Geometry check sheet. Reference: the model listing, model coordinates, mm. Round coordinates to 2 decimals unless told otherwise and drop trailing zeros. Loops run counter-clockwise (first coordinate to the right, second up) from the corner with the lowest first, then second, coordinate; pieces in that order, holes last. Notation, with made-up numbers: (63, 35.5) -> (90, 35.5) arc R29 ccw to (90, 65.5) -> close; hole circle Ø7 at (59, 22). An arc over 180 degrees is marked (long way). Use a Markdown table: item, result. Add a question column.
Q1. Gauge pin test, flat end, axial feed: P1, Ø1, axis at x = 0.5, z = 2.5, coming from the -Y side. Record the tip position at first contact, or that the pin passes through.
Q2. Sectioned sample at B-B, the plane x = 4.5. Enter the section's corners in (y, z).
Q3. Sectioned sample at A-A, the plane y = -6. Enter the section's corners in (x, z).
Q4. Material ranges on L1, parallel to Y at x = 2.75, z = 2.2; L2, parallel to X at y = -1.5, z = 4.25, recorded low to high.
```python
from build123d import *

# Parameters (mm, degrees)
F0_R     = 10
F1_DEPTH = 5


with BuildPart() as f1:
    # F0 (on Top) → F1 (new body)
    with BuildSketch(Plane.XY):
        Circle(F0_R)
        Polygon((-0.372, 2.825618), (0, 2.540172), (0.372, 2.825618), (0.657445, 2.453618), (1.090648, 2.633057), (1.270086, 2.199854), (1.73497, 2.261057), (1.796173, 1.796173), (2.261057, 1.73497), (2.199854, 1.270086), (2.633057, 1.090648), (2.453618, 0.657445), (2.825618, 0.372), (2.540172, 0), (2.825618, -0.372), (2.453618, -0.657445), (2.633057, -1.090648), (2.199854, -1.270086), (2.261057, -1.73497), (1.796173, -1.796173), (1.73497, -2.261057), (1.270086, -2.199854), (1.090648, -2.633057), (0.657445, -2.453618), (0.372, -2.825618), (0, -2.540172), (-0.372, -2.825618), (-0.657445, -2.453618), (-1.090648, -2.633057), (-1.270086, -2.199854), (-1.73497, -2.261057), (-1.796173, -1.796173), (-2.261057, -1.73497), (-2.199854, -1.270086), (-2.633057, -1.090648), (-2.453618, -0.657445), (-2.825618, -0.372), (-2.540172, 0), (-2.825618, 0.372), (-2.453618, 0.657445), (-2.633057, 1.090648), (-2.199854, 1.270086), (-2.261057, 1.73497), (-1.796173, 1.796173), (-1.73497, 2.261057), (-1.270086, 2.199854), (-1.090648, 2.633057), (-0.657445, 2.453618), align=None, mode=Mode.SUBTRACT)
    extrude(amount=F1_DEPTH)


solid = f1.part
```
Values:
| question | item | result |
|---|---|---|
| 1 | P1 | y = -10 |
| 2 | outline | (-8.93, 0) -> (8.93, 0) -> (8.93, 5) -> (-8.93, 5) -> close |
| 3 | outline | (-8, 0) -> (8, 0) -> (8, 5) -> (-8, 5) -> close |
| 4 | L1 | -9.61 to -0.43, -0.27 to 0.27, 0.43 to 9.61 |
| 4 | L2 | -9.89 to -2.23, 2.23 to 9.89 |
